from build123d import *

# Parameters (mm, degrees)
F0_W      = 145
F0_H      = 50
F1_DEPTH  = 5
F2_R      = 2.5
F2_R_2    = 1.5
F3_DEPTH  = 9.75
F4_R      = 1.5
F5_DEPTH  = 25
F6_W      = 5
F6_H      = 45
F7_DEPTH  = 145
F9_DEPTH  = 5
F10_START = -70
F10_DEPTH = 5
F11_START = -140
F11_DEPTH = 5
F12_R     = 2.5
F12_R_2   = 1.5
F13_DEPTH = 5


with BuildPart() as f1:
    # F0 (on Top) → F1 (new body)
    with BuildSketch(Plane.XY):
        with Locations((72.5, 25)):
            Rectangle(F0_W, F0_H)
    extrude(amount=F1_DEPTH)

    # F2 (on face) → F3 (join)
    with BuildSketch(Plane.XY.offset(5)):
        with Locations((20, 42.5)):
            Circle(F2_R)
        with Locations((20, 42.5)):
            Circle(F2_R_2, mode=Mode.SUBTRACT)
        with Locations((20, 22.04)):
            Circle(F2_R)
        with Locations((20, 22.04)):
            Circle(F2_R_2, mode=Mode.SUBTRACT)
        with Locations((125, 42.5)):
            Circle(F2_R)
        with Locations((125, 42.5)):
            Circle(F2_R_2, mode=Mode.SUBTRACT)
        with Locations((125, 22.04)):
            Circle(F2_R)
        with Locations((125, 22.04)):
            Circle(F2_R_2, mode=Mode.SUBTRACT)
    extrude(amount=F3_DEPTH)

    # F4 (on face) → F5 (cut)
    with BuildSketch(Plane.XY.offset(5)):
        with Locations((20, 42.5)):
            Circle(F4_R)
        with Locations((20, 22.04)):
            Circle(F4_R)
        with Locations((125, 42.5)):
            Circle(F4_R)
        with Locations((125, 22.04)):
            Circle(F4_R)
    extrude(amount=-F5_DEPTH, mode=Mode.SUBTRACT)

    # F6 (on face) → F7 (join, through all)
    with BuildSketch(Plane.YZ.offset(145)):
        with Locations((47.5, -22.5)):
            Rectangle(F6_W, F6_H)
    extrude(amount=-F7_DEPTH)

    # F8 (on face) → F9 (join)
    with BuildSketch(Plane(origin=(0, 0, 0), x_dir=(0, -1, 0), z_dir=(-1, 0, 0))):
        Polygon((-45, 0), (-45, -45), (0, 0), align=None)
    extrude(amount=-F9_DEPTH)

    # F8 (on face) → F10 (join)
    with BuildSketch(Plane(origin=(0, 0, 0), x_dir=(0, -1, 0), z_dir=(-1, 0, 0)).offset(F10_START)):
        Polygon((-45, 0), (-45, -45), (0, 0), align=None)
    extrude(amount=-F10_DEPTH)

    # F8 (on face) → F11 (join)
    with BuildSketch(Plane(origin=(0, 0, 0), x_dir=(0, -1, 0), z_dir=(-1, 0, 0)).offset(F11_START)):
        Polygon((-45, 0), (-45, -45), (0, 0), align=None)
    extrude(amount=-F11_DEPTH)

    # F12 (on face) → F13 (join)
    with BuildSketch(Plane(origin=(0, 50, 0), x_dir=(-1, 0, 0), z_dir=(0, 1, 0))):
        with Locations((-102.5, -5)):
            Circle(F12_R)
        with Locations((-102.5, -5)):
            Circle(F12_R_2, mode=Mode.SUBTRACT)
        with Locations((-102.5, -25.46)):
            Circle(F12_R)
        with Locations((-102.5, -25.46)):
            Circle(F12_R_2, mode=Mode.SUBTRACT)
        with Locations((-42.5, -5)):
            Circle(F12_R)
        with Locations((-42.5, -5)):
            Circle(F12_R_2, mode=Mode.SUBTRACT)
        with Locations((-42.5, -25.46)):
            Circle(F12_R)
        with Locations((-42.5, -25.46)):
            Circle(F12_R_2, mode=Mode.SUBTRACT)
    extrude(amount=F13_DEPTH)


solid = f1.part
Input: part model. Units: mm. Frame: model coordinates. A direction names the side the tool comes from. Give positions to 0.01 mm unless a question says otherwise; leave off trailing zeros. Write each loop counter-clockwise with the first axis right and the second up, starting at its lowest first coordinate (ties: lowest second). Pieces come first, ordered by that corner, then holes. Notation, with made-up numbers: (11.25, -17.5) -> (31.25, -17.5) arc R21 cw to (31.25, 6.5) -> close; hole circle Ø6 at (69.5, 24). An arc over 180 degrees is marked (long way). Use one line per item in the form item = value. Start each with the question number.
1) Set-up query: faces 1 (the flat face through (126, 41, 14.75)), 2 (the flat face through (38, 45, -23)), 3 (the cylindrical face through (40.19, 52.46, -5.96)). Return all of +Z, -Z, +X, -X, +Y, -Y with unobstructed straight access to the full face (end or side cutting, diameter ignored); none if empty.
2) Section query A-A on y = 42.5. Return the cut outline in (x, z).
3) Draft query along X for faces 4 (the cylindrical face through (127.385, 43.251, 9.807)), 5 (the flat face through (71, 0, 2)), 6 (the flat face through (0, 31, -14)). Return one class per face: pulls with the +X half, pulls with the -X half, needs draft (parallel to the pull), parting line crosses it, or undercut.
4) Section query D-D on y = 22.04. Return the cut outline in (x, z).
5) Ray query, probe 1 along Z at (x, y) = (42.5, 51.5); probe 2 along X at (y, z) = (39.5, -13); probe 3 along X at (y, z) = (22, 2). Return the intervals inside material, ascending. Write a range as from..to.
6) Pin query (flat end, axial travel): pin 1 (10 mm diameter, centred on x = 52.5, z = -24, fed in from +Y); pin 2 (13.5 mm diameter, centred on x = 101, y = 19, fed in from -Z); pin 3 (2 mm diameter, centred on x = 55, y = 44.5, fed in from +Z). Return the tip coordinate at first contact, or that it passes through.
7) Section query C-C on x = 20. Return the cut outline in (y, z).
8) Section query B-B on z = 8. Return the cut outline in (x, y), then the cut area to 3 significant figures.
Outcome:
q1.face_1 = +Z, +X, -X, +Y, -Y
q1.face_2 = -Z, -Y
q1.face_3 = +Y
q2.outline = (0, -42.5) -> (5, -42.5) -> (5, 0) -> (18.5, 0) -> (18.5, 14.75) -> (17.5, 14.75) -> (17.5, 5) -> (0, 5) -> close; (21.5, 0) -> (70, 0) -> (70, -42.5) -> (75, -42.5) -> (75, 0) -> (123.5, 0) -> (123.5, 14.75) -> (122.5, 14.75) -> (122.5, 5) -> (22.5, 5) -> (22.5, 14.75) -> (21.5, 14.75) -> close; (126.5, 0) -> (140, 0) -> (140, -42.5) -> (145, -42.5) -> (145, 5) -> (127.5, 5) -> (127.5, 14.75) -> (126.5, 14.75) -> close
q3.face_4 = undercut
q3.face_5 = needs draft
q3.face_6 = pulls with the -X half
q4.outline = (0, -22.04) -> (5, -22.04) -> (5, 0) -> (18.5, 0) -> (18.5, 14.75) -> (17.5, 14.75) -> (17.5, 5) -> (0, 5) -> close; (21.5, 0) -> (70, 0) -> (70, -22.04) -> (75, -22.04) -> (75, 0) -> (123.5, 0) -> (123.5, 14.75) -> (122.5, 14.75) -> (122.5, 5) -> (22.5, 5) -> (22.5, 14.75) -> (21.5, 14.75) -> close; (126.5, 0) -> (140, 0) -> (140, -22.04) -> (145, -22.04) -> (145, 5) -> (127.5, 5) -> (127.5, 14.75) -> (126.5, 14.75) -> close
q5.probe_1 = -27.96..-26.96, -23.96..-22.96, -7.5..-6.5, -3.5..-2.5
q5.probe_2 = 0..5, 70..75, 140..145
q5.probe_3 = 0..18.5, 21.5..123.5, 126.5..145
q6.pin_1 = 50
q6.pin_2 = 0
q6.pin_3 = 5
q7.outline = (0, 0) -> (20.54, 0) -> (20.54, 14.75) -> (19.54, 14.75) -> (19.54, 5) -> (0, 5) -> close; (23.54, 0) -> (41, 0) -> (41, 14.75) -> (40, 14.75) -> (40, 5) -> (24.54, 5) -> (24.54, 14.75) -> (23.54, 14.75) -> close; (44, 0) -> (45, 0) -> (45, -45) -> (50, -45) -> (50, 5) -> (45, 5) -> (45, 14.75) -> (44, 14.75) -> close
q8.outline = circle Ø5 at (20, 22.04); circle Ø5 at (20, 42.5); circle Ø5 at (125, 22.04); circle Ø5 at (125, 42.5); hole circle Ø3 at (20, 22.04); hole circle Ø3 at (20, 42.5); hole circle Ø3 at (125, 22.04); hole circle Ø3 at (125, 42.5)
q8.area = 50.3 mm^2
